Geometry: final body of the model. Coordinates: model frame, mm. A direction names the side the tool comes from. Round coordinates to 2 decimals unless told otherwise and drop trailing zeros. Order: outer loops, then holes, each group sorted by start corner. A loop starts at its lowest first (then second) coordinate and runs counter-clockwise, first axis right, second up. Notation, with made-up numbers: M 77,28 L 121,28 A20 ccw 121,62 Z; hole C 28.5,77 d10. An arc over 180 degrees is marked long. Put each result on its own line as item: value. Start each with the question number.
1) Section C-C, the plane z = 60.5. Return loops of the section in (x, y), then the cut area to 3 significant figures.
2) Section B-B, the plane y = 30. Return loops of the section in (x, z), then the cut area to 3 significant figures.
3) First-contact query: P1, Ø0.5, axis at x = 0.5, z = 8.5, coming from the -Y side; P2, Ø3.5, axis at x = 4.5, y = 1.5, coming from the +Z side; P3, Ø1, axis at x = 10, z = 76, coming from the +Y side. Flat tips, straight axial feed; report the tip coordinate or a pass-through.
4) Section D-D, the plane z = 328. Return loops of the section in (x, y).
5) Access query for faces 1 (the flat face through (1, 21, 168)), 2 (the cylindrical face through (0.493, 31.892, 175.936)). Directions: +Z, -Z, +X, -X, +Y, -Y. A direction counts if a zero-diameter tool reaches every point of the face in a straight line with its end or side. Return the directions, or none.
6) Section A-A, the plane z = 178. Return loops of the section in (x, y).
7) Material intervals for probe 1 along Z at (x, y) = (11, 0.4); probe 2 along Y at (x, z) = (10.75, 219), sorted ascending. Write a range as [from, to].
8) Draft query along Z for faces 3 (the cylindrical face through (0.5, 30.1, 325.2)), 4 (the flat face through (9, 1, 168)), 5 (the cylindrical face through (0.493, 31.892, 25.936)). Return one class per face: pulls with the +Z half, pulls with the -Z half, needs draft (parallel to the pull), parting line crosses it, or undercut.
from build123d import *

# Parameters (mm, degrees)
EXTRUDE_1_DEPTH     = 340
SKETCH_2_R          = 2.8
CUT_EXTRUDE_1_DEPTH = 340
SKETCH_3_R          = 2.15
CUT_EXTRUDE_2_DEPTH = 340
SKETCH_4_W          = 37.623292197
SKETCH_4_H          = 20.655925128
SKETCH_4_W_2        = 42.547460075
SKETCH_4_H_2        = 15
CUT_EXTRUDE_3_DEPTH = 3


with BuildPart() as part:
    # Эскиз1 → Вытянуть1 (new body)
    with BuildSketch(Plane.XY):
        with BuildLine():
            Line((17, 0), (2, 0))
            ThreePointArc((2, 0), (0.585786438, 0.585786438), (0, 2))
            Line((0, 2), (0, 40))
            Line((0, 40), (1, 40))
            Line((1, 40), (1, 2))
            ThreePointArc((1, 2), (1.292893219, 1.292893219), (2, 1))
            Line((2, 1), (17, 1))
            Line((17, 1), (17, 0))
        make_face()
    extrude(amount=EXTRUDE_1_DEPTH)

    # Эскиз2 → Вырез-Вытянуть1 (cut)
    with BuildSketch(Plane.ZY):
        with Locations((28, 30)):
            Circle(SKETCH_2_R)
        with Locations((178, 30)):
            Circle(SKETCH_2_R)
        with Locations((328, 30)):
            Circle(SKETCH_2_R)
    extrude(amount=-CUT_EXTRUDE_1_DEPTH, mode=Mode.SUBTRACT)

    # Эскиз3 → Вырез-Вытянуть2 (cut)
    with BuildSketch(Plane.XZ):
        with Locations((11, 30)):
            Circle(SKETCH_3_R)
        with Locations((11, 100)):
            Circle(SKETCH_3_R)
        with Locations((11, 170)):
            Circle(SKETCH_3_R)
        with Locations((11, 240)):
            Circle(SKETCH_3_R)
    extrude(amount=-CUT_EXTRUDE_2_DEPTH, mode=Mode.SUBTRACT)

    # Эскиз4 → Вырез-Вытянуть3 (cut)
    with BuildSketch(Plane.XZ):
        with Locations((6.462024168, 335.327962564)):
            Rectangle(SKETCH_4_W, SKETCH_4_H)
        with Locations((3.999940229, 7.5)):
            Rectangle(SKETCH_4_W_2, SKETCH_4_H_2)
    extrude(amount=-CUT_EXTRUDE_3_DEPTH, mode=Mode.SUBTRACT)


solid = part.part
Result sheet:
1. outline: M 0,2 A2 ccw 2,0 L 17,0 L 17,1 L 2,1 A1 cw 1,2 L 1,40 L 0,40 Z
1. area: 55.4 mm2
2. outline: M 0,0 L 1,0 L 1,25.2 L 0,25.2 Z; M 0,30.8 L 1,30.8 L 1,175.2 L 0,175.2 Z; M 0,180.8 L 1,180.8 L 1,325.2 L 0,325.2 Z; M 0,330.8 L 1,330.8 L 1,340 L 0,340 Z
2. area: 323 mm2
3. P1: stops at y = 3
3. P2: stops at z = 325
3. P3: stops at y = 1
4. outline: M 0,3 L 1,3 L 1,27.2 L 0,27.2 Z; M 0,32.8 L 1,32.8 L 1,40 L 0,40 Z
5. face 1: +Z, -Z, +X, +Y
5. face 2: +X, -X
6. outline: M 0,2 A2 ccw 2,0 L 17,0 L 17,1 L 2,1 A1 cw 1,2 L 1,27.2 L 0,27.2 Z; M 0,32.8 L 1,32.8 L 1,40 L 0,40 Z
7. probe 1: z = [15, 27.85], [32.15, 97.85], [102.15, 167.85], [172.15, 237.85], [242.15, 325]
7. probe 2: y = [0, 1]
8. face 3: undercut
8. face 4: needs draft
8. face 5: undercut
